Check sheet for the modelled part. Datum: model origin and axes. Units: mm. Face numbers are marked on the shaded views. Round coordinates to 2 decimals unless told otherwise and drop trailing zeros. Write each loop counter-clockwise with the first axis right and the second up, starting at its lowest first coordinate (ties: lowest second). Pieces come first, ordered by that corner, then holes.
Item 1: Cross-section at B-B on z = -28.5. Enter the section's corners in (x, y).
Item 2: Cross-section at A-A on x = 2.3. Enter the section's corners in (y, z).
Item 3: Material ranges on line 1 (Z direction, x = 40.9, y = 1.1); line 2 (X direction, y = 0.5, z = -3.5); line 3 (X direction, y = 5.25, z = -20.5), recorded low to high.
Item 4: Cross-section at C-C on y = 3.25. Enter the section's corners in (x, z), plus the area to 3 significant figures.
Item 5: Release check for a two-part mould opening along Z. For the marked faces 1, 2 and 3 record: +Z half, -Z half, draft (parallel to the pull), parting line (faces both ways), or undercut.
Item 6: Cross-section at D-D on x = 48. Enter the section's corners in (y, z), plus the area to 3 significant figures.
Item 7: Go/stop test with flat-tipped pins: pin 1 Ø1.5 at (x, y) = (68, 7) entering from +Z; pin 2 Ø2 at (x, y) = (37.5, 6) entering from -Z; pin 3 Ø0.7 at (x, z) = (28.2, -33.65) entering from -Y; pin 4 Ø1.4 at (x, z) = (45.98, -33.65) entering from +Y. Record where each tip stops, or that it passes through.
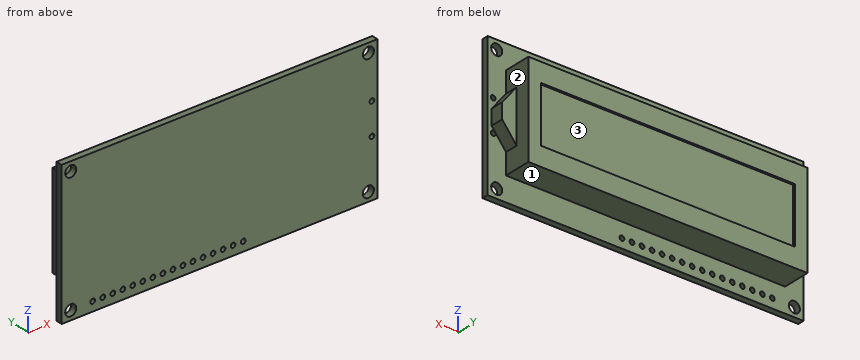
from build123d import *

# Parameters (mm, degrees)
SKETCH1_W           = 80
SKETCH1_H           = 36
SKETCH1_R           = 1.4
BOSS_EXTRUDE1_DEPTH = 1.6
SKETCH2_W           = 70.7
SKETCH2_H           = 23.8
BOSS_EXTRUDE2_DEPTH = 7
SKETCH3_W           = 64.3
SKETCH3_H           = 14.2
CUT_EXTRUDE1_DEPTH  = 0.5
BOSS_EXTRUDE3_DEPTH = 3.3
SKETCH5_R           = 0.6
CUT_EXTRUDE2_DEPTH  = 2.6


with BuildPart() as part:
    # Sketch1 → Boss-Extrude1 (new body)
    with BuildSketch(Plane(origin=(0, 0, 0), x_dir=(1, 0, 0), z_dir=(0, 1, 0))):
        with Locations((40, 18)):
            Rectangle(SKETCH1_W, SKETCH1_H)
        with Locations((2.3, 33.711820065)):
            Circle(SKETCH1_R, mode=Mode.SUBTRACT)
        with Locations((2.3, 2.288179935)):
            Circle(SKETCH1_R, mode=Mode.SUBTRACT)
        with Locations((77.7, 2.288179935)):
            Circle(SKETCH1_R, mode=Mode.SUBTRACT)
        with Locations((77.7, 33.711820065)):
            Circle(SKETCH1_R, mode=Mode.SUBTRACT)
    extrude(amount=BOSS_EXTRUDE1_DEPTH)

    # Sketch2 → Boss-Extrude2 (add)
    with BuildSketch(Plane(origin=(0, 1.6, 0), x_dir=(1, 0, 0), z_dir=(0, 1, 0))):
        with Locations((40, 18)):
            Rectangle(SKETCH2_W, SKETCH2_H)
    extrude(amount=BOSS_EXTRUDE2_DEPTH)

    # Sketch3 → Cut-Extrude1 (cut)
    with BuildSketch(Plane(origin=(0, 8.6, 0), x_dir=(1, 0, 0), z_dir=(0, 1, 0))):
        with Locations((40, 18)):
            Rectangle(SKETCH3_W, SKETCH3_H)
    extrude(amount=-CUT_EXTRUDE1_DEPTH, mode=Mode.SUBTRACT)

    # Sketch4 → Boss-Extrude3 (add)
    with BuildSketch(Plane(origin=(0, 1.6, 0), x_dir=(1, 0, 0), z_dir=(0, 1, 0))):
        Polygon((75.35, 24.6), (79, 19.94), (79, 16.06), (75.35, 11.4), align=None)
    extrude(amount=BOSS_EXTRUDE3_DEPTH)

    # Sketch5 → Cut-Extrude2 (cut, through all)
    with BuildSketch(Plane(origin=(0, 1.6, 0), x_dir=(1, 0, 0), z_dir=(0, 1, 0))):
        with Locations((7.88, 33.65)):
            Circle(SKETCH5_R)
        with Locations((10.42, 33.65)):
            Circle(SKETCH5_R)
        with Locations((12.96, 33.65)):
            Circle(SKETCH5_R)
        with Locations((15.5, 33.65)):
            Circle(SKETCH5_R)
        with Locations((18.04, 33.65)):
            Circle(SKETCH5_R)
        with Locations((20.58, 33.65)):
            Circle(SKETCH5_R)
        with Locations((23.12, 33.65)):
            Circle(SKETCH5_R)
        with Locations((25.66, 33.65)):
            Circle(SKETCH5_R)
        with Locations((28.2, 33.65)):
            Circle(SKETCH5_R)
        with Locations((30.74, 33.65)):
            Circle(SKETCH5_R)
        with Locations((33.28, 33.65)):
            Circle(SKETCH5_R)
        with Locations((35.82, 33.65)):
            Circle(SKETCH5_R)
        with Locations((38.36, 33.65)):
            Circle(SKETCH5_R)
        with Locations((40.9, 33.65)):
            Circle(SKETCH5_R)
        with Locations((43.44, 33.65)):
            Circle(SKETCH5_R)
        with Locations((45.98, 33.65)):
            Circle(SKETCH5_R)
        with Locations((78.6, 21.5)):
            Circle(SKETCH5_R)
        with Locations((78.6, 13.5)):
            Circle(SKETCH5_R)
    extrude(amount=-CUT_EXTRUDE2_DEPTH, mode=Mode.SUBTRACT)


solid = part.part
Response values:
1. outline: (0, 0) - (80, 0) - (80, 1.6) - (75.35, 1.6) - (75.35, 8.6) - (4.65, 8.6) - (4.65, 1.6) - (0, 1.6) - close
2. outline: (0, -36) - (1.6, -36) - (1.6, -35.11) - (0, -35.11) - close; (0, -32.31) - (1.6, -32.31) - (1.6, -3.69) - (0, -3.69) - close; (0, -0.89) - (1.6, -0.89) - (1.6, 0) - (0, 0) - close
3. line 1: z = -36 to -34.25, -33.05 to 0
3. line 2: x = 0 to 1.6, 3 to 77, 78.4 to 80
3. line 3: x = 4.65 to 75.35
4. outline: (4.65, -29.9) - (75.35, -29.9) - (75.35, -24.6) - (79, -19.94) - (79, -16.06) - (75.35, -11.4) - (75.35, -6.1) - (4.65, -6.1) - close
4. area: 1,710 mm2
5. face 1: -Z half
5. face 2: draft
5. face 3: undercut
6. outline: (0, -36) - (1.6, -36) - (1.6, -29.9) - (8.6, -29.9) - (8.6, -25.1) - (8.1, -25.1) - (8.1, -10.9) - (8.6, -10.9) - (8.6, -6.1) - (1.6, -6.1) - (1.6, 0) - (0, 0) - close
6. area: 217 mm2
7. pin 1: stops at z = -6.1
7. pin 2: stops at z = -29.9
7. pin 3: passes through
7. pin 4: stops at y = 1.6
